```python
from build123d import *

# Parameters (mm, degrees)
F1_DEPTH = 20.87
F2_W     = 6
F2_H     = 8
F2_W_2   = 1
F2_H_2   = 10
F4_R     = 0.5
F5_R     = 1


with BuildPart() as f1:
    # F0 (on Front) → F1 (new body, symmetric)
    with BuildSketch(Plane.XZ):
        Polygon((-21, 6.1), (-12.9, 6.1), (0, 6.1), (0, 11), (-6, 11), (-7, 11), (-21, 11), align=None)
        Polygon((0, 11), (0, 6.1), (12.9, 6.1), (21, 6.1), (21, 11), (7, 11), (6, 11), align=None)
        Polygon((-12.9, 6.1), (-19, 0), (0, 0), (19, 0), (12.9, 6.1), (0, 6.1), align=None)
    extrude(amount=F1_DEPTH, both=True)

    # F2 (on Front) → F3 (revolve)
    with BuildSketch(Plane.XZ):
        with Locations((-3, 15)):
            Rectangle(F2_W, F2_H)
        with Locations((-6.5, 15)):
            Rectangle(F2_W_2, F2_H)
        with Locations((-3, 24)):
            Rectangle(F2_W, F2_H_2)
    revolve(axis=Axis((0, 0, 20), (0, 0, -1)))

    # F4
    f4_edges = [f1.edges().sort_by_distance(p)[0] for p in [
        (6, 0, 29),
        (7, 0, 19),
    ]]
    fillet(f4_edges, radius=F4_R)

    # F5
    f5_edges = [f1.edges().sort_by_distance(p)[0] for p in [
        (-21, 0, 11),
        (0, -20.87, 11),
        (0, 20.87, 11),
        (21, 0, 11),
        (7, 0, 11),
        (-21, 20.87, 8.55),
        (-21, 0, 6.1),
        (-21, -20.87, 8.55),
        (21, 0, 6.1),
        (21, 20.87, 8.55),
        (21, -20.87, 8.55),
        (16.95, 20.87, 6.1),
        (-16.95, 20.87, 6.1),
        (-16.95, -20.87, 6.1),
        (16.95, -20.87, 6.1),
    ]]
    fillet(f5_edges, radius=F5_R)


solid = f1.part
```
Read the model definition and answer for the solid it produces. Units are mm, in the model's axes. A direction names the side the tool comes from. Round coordinates to 2 decimals unless told otherwise and drop trailing zeros. Loops run counter-clockwise (first coordinate to the right, second up) from the corner with the lowest first, then second, coordinate; pieces in that order, holes last. Notation, with made-up numbers: (-27.5, -17) -> (27.5, -17) arc R16 cw to (27.5, -7) -> close; hole circle Ø8 at (-40, 33.25). An arc over 180 degrees is marked (long way). One line per item, written item: value.
1) A cutting plane is placed at D-D (z = 5). Determine the outline of the cut face in (x, y), and give its area (3 significant figures).
Answer list:
outline: (-14, -20.87) -> (14, -20.87) -> (14, 20.87) -> (-14, 20.87) -> close
area: 1,170 mm²
2) A cutting plane is placed at B-B (x = 0). Determine the outline of the cut face in (y, z).
Answer list:
outline: (-20.87, 0) -> (20.87, 0) -> (20.87, 10) arc R1 ccw to (19.87, 11) -> (8, 11) arc R1 cw to (7, 12) -> (7, 18.5) arc R0.5 ccw to (6.5, 19) -> (6, 19) -> (6, 28.5) arc R0.5 ccw to (5.5, 29) -> (-5.5, 29) arc R0.5 ccw to (-6, 28.5) -> (-6, 19) -> (-6.5, 19) arc R0.5 ccw to (-7, 18.5) -> (-7, 12) arc R1 cw to (-8, 11) -> (-19.87, 11) arc R1 ccw to (-20.87, 10) -> close
3) Consider L1, parallel to Z at x = 9, y = 9; L2, parallel to Z at x = 13.5, y = 1; L3, parallel to Z at x = -18.5, y = 11. Determine where each line is inside the solid, lowest interval first. Write a range as [from, to].
Answer list:
L1: z = [0, 11]
L2: z = [0, 5.5], [6.1, 11]
L3: z = [0, 0.5], [6.1, 11]
4) A cutting plane is placed at A-A (x = 16). Determine the outline of the cut face in (y, z), and give its area (3 significant figures).
Answer list:
outline: (-20.87, 0) -> (20.87, 0) -> (20.87, 3) -> (-20.87, 3) -> close; (-20.87, 7.1) arc R1 ccw to (-19.87, 6.1) -> (19.87, 6.1) arc R1 ccw to (20.87, 7.1) -> (20.87, 10) arc R1 ccw to (19.87, 11) -> (-19.87, 11) arc R1 ccw to (-20.87, 10) -> close
area: 329 mm²
5) Flat-ended cylindrical pins translate along their axes: P1, Ø2, axis at x = 2, y = -7, coming from the +Z side; P2, Ø4, axis at y = 10, z = 3.5, coming from the -X side; P3, Ø4, axis at x = -6.5, z = 16.5, coming from the -Y side. Find the tip coordinate at first contact, or state that the pin passes through.
Answer list:
P1: stops at z = 19
P2: stops at x = -17.5
P3: stops at y = -5.36
6) A cutting plane is placed at C-C (y = 0). Determine the outline of the cut face in (x, z), and give its area (3 significant figures).
Answer list:
outline: (-21, 7.1) arc R1 ccw to (-20, 6.1) -> (-12.9, 6.1) -> (-19, 0) -> (19, 0) -> (12.9, 6.1) -> (20, 6.1) arc R1 ccw to (21, 7.1) -> (21, 10) arc R1 ccw to (20, 11) -> (8, 11) arc R1 cw to (7, 12) -> (7, 18.5) arc R0.5 ccw to (6.5, 19) -> (6, 19) -> (6, 28.5) arc R0.5 ccw to (5.5, 29) -> (-5.5, 29) arc R0.5 ccw to (-6, 28.5) -> (-6, 19) -> (-6.5, 19) arc R0.5 ccw to (-7, 18.5) -> (-7, 12) arc R1 cw to (-8, 11) -> (-20, 11) arc R1 ccw to (-21, 10) -> close
area: 632 mm²
7) The mould has two halves that part along Z. Classify faces 5 (the face through (-0.28, -20.569, 10.715)), 6 (the face through (-16, 0, 6.1)), 7 (the face through (0, -20.87, 5)): pulls with the +Z half, pulls with the -Z half, needs draft (parallel to the pull), parting line crosses it, or undercut.
Answer list:
face 5: pulls with the +Z half
face 6: undercut
face 7: needs draft
8) For faces 1 (the face through (-15.893, -20.585, 6.401)), 2 (the face through (16, 0, 6.1)), 3 (the face through (0, 9, 11)), 4 (the face through (-15.893, 20.585, 6.401)), determine the directions among +Z, -Z, +X, -X, +Y, -Y from which every point of the face is accessible in a straight line to the end or side of a thin tool.
Answer list:
face 1: -X, -Y
face 2: +X, +Y, -Y
face 3: +Z
face 4: -X, +Y
